from build123d import *

# Parameters (mm, degrees)
SKETCH1_R           = 5
BOSS_EXTRUDE1_DEPTH = 6
BOSS_EXTRUDE2_DEPTH = 3
SKETCH3_R           = 3
SKETCH3_R_2         = 1.25
CUT_EXTRUDE1_DEPTH  = 14.865424624
FILLET1_R           = 0.3
CHAMFER1_SIZE       = 0.1


with BuildPart() as part:
    # Sketch1 → Boss-Extrude1 (new body)
    with BuildSketch(Plane.XY):
        Circle(SKETCH1_R)
    extrude(amount=BOSS_EXTRUDE1_DEPTH)

    # Sketch2 → Boss-Extrude2 (add)
    with BuildSketch(Plane(origin=(0, 0, 0), x_dir=(-1, 0, 0), z_dir=(0, 0, -1))):
        with BuildLine():
            Line((-4.763139721, 2.75), (-1.732050808, 8))
            ThreePointArc((-1.732050808, 8), (0, 9), (1.732050808, 8))
            Line((1.732050808, 8), (4.763139721, 2.75))
            ThreePointArc((4.763139721, 2.75), (5.5, 0), (4.763139721, -2.75))
            Line((4.763139721, -2.75), (1.732050808, -8))
            ThreePointArc((1.732050808, -8), (0, -9), (-1.732050808, -8))
            Line((-1.732050808, -8), (-4.763139721, -2.75))
            ThreePointArc((-4.763139721, -2.75), (-5.5, 0), (-4.763139721, 2.75))
        make_face()
    extrude(amount=BOSS_EXTRUDE2_DEPTH)

    # Sketch3 → Cut-Extrude1 (cut, through all)
    with BuildSketch(Plane(origin=(0, 0, -3), x_dir=(-1, 0, 0), z_dir=(0, 0, -1))):
        Circle(SKETCH3_R)
        with Locations((0, 7)):
            Circle(SKETCH3_R_2)
        with Locations((0, -7)):
            Circle(SKETCH3_R_2)
    extrude(amount=-CUT_EXTRUDE1_DEPTH, mode=Mode.SUBTRACT)

    # Fillet1
    fillet1_edges = [part.edges().sort_by_distance(p)[0] for p in [
        (-5, 0, 0),
    ]]
    fillet(fillet1_edges, radius=FILLET1_R)

    # Chamfer1
    chamfer1_edges = [part.edges().sort_by_distance(p)[0] for p in [
        (-3.247595264, -5.375, -3),
        (-5.5, 0, -3),
        (-3.247595264, 5.375, -3),
        (0, 9, -3),
        (3.247595264, 5.375, -3),
        (1.25, -7, 0),
        (1.25, -7, -3),
        (1.25, 7, 0),
        (1.25, 7, -3),
        (3, 0, 6),
        (3, 0, -3),
        (-5, 0, 6),
        (5.5, 0, 0),
        (3.247595264, -5.375, 0),
        (0, -9, 0),
        (-3.247595264, -5.375, 0),
        (-5.5, 0, 0),
        (-3.247595264, 5.375, 0),
        (0, 9, 0),
        (3.247595264, 5.375, 0),
        (5.5, 0, -3),
        (3.247595264, -5.375, -3),
        (0, -9, -3),
    ]]
    chamfer(chamfer1_edges, length=CHAMFER1_SIZE)


solid = part.part
Part model, mm, in its own coordinate system. A direction names the side the tool comes from. Coordinates: 2 decimals unless noted, no trailing zeros. Loops run counter-clockwise (first coordinate to the right, second up) from the corner with the lowest first, then second, coordinate; pieces in that order, holes last. Notation, with made-up numbers: M 76,65 L 96,65 A29 cw 96,102 Z; hole C -5.5,85 d11. An arc over 180 degrees is marked long. Use a Markdown table: item, result. Add a question column.
Q1. Probe L1, parallel to Y at x = 0, z = 3; L2, parallel to Z at x = -2.25, y = 5.25; L3, parallel to Y at x = -1, z = -0.5. List the from-to ranges inside material, lowest first.
Q2. Pin check, flat tips, straight feed: P1, Ø3, axis at x = -2.5, z = 3.5, coming from the -Y side; P2, Ø4, axis at x = -4, y = -7, coming from the +Z side; P3, Ø2, axis at x = 3, z = 4.5, coming from the -Y side. Stop position of each tip, or through.
Q3. Cut at B-B (z = -2). Write the cut outline in (x, y), and give its area (3 significant figures).
Q4. Cut at D-D (x = 0). Give the number of separate pieces and of enclosed holes in the cut face, and give its area (3 significant figures).
Q5. Which spindle directions (+Z, -Z, +X, -X, +Y, -Y) get a long thin tool onto all of the face, cutting with end or side? Do faces 1 (the flat face through (3.226, -5.412, -1.48)), 2 (the cylindrical face through (-1.08, -4.88, 3.06)). Say none if no direction does.
Q6. Cut at C-C (z = 3.75). Write the cut outline in (x, y).
Q7. Cut at A-A (y = 0). Write the cut outline in (x, z), and give its area (3 significant figures).
Q8. Mould opens along Y. For faces 3 (the cylindrical face through (0.27, 5.78, -1.52)), 4 (the cylindrical face through (-5.5, 0, -1.5)), 5 (the flat face through (-3.27, -5.34, -1.48)) say: +Y half, -Y half, draft (parallel to the pull), parting line (faces both ways), or undercut.
Worked out:
| question | item | result |
|---|---|---|
| 1 | L1 | y = -5 to -3, 3 to 5 |
| 1 | L2 | z = -3 to 0 |
| 1 | L3 | y = -8.73 to -7.75, -6.25 to -2.83, 2.83 to 6.25, 7.75 to 8.73 |
| 2 | P1 | stops at y = -4.9 |
| 2 | P2 | stops at z = 0 |
| 2 | P3 | stops at y = -4.58 |
| 3 | outline | M -4.76,-2.75 L -1.73,-8 A2 ccw 1.73,-8 L 4.76,-2.75 A5.5 ccw 4.76,2.75 L 1.73,8 A2 ccw -1.73,8 L -4.76,2.75 A5.5 ccw Z; hole C 0,0 d6; hole C 0,-7 d2.5; hole C 0,7 d2.5 |
| 3 | area | 92.9 mm2 |
| 4 | separate pieces | 4 |
| 4 | enclosed holes | 0 |
| 4 | area | 44.9 mm2 |
| 5 | face 1 | +Z, -Z, +X, -Y |
| 5 | face 2 | +Z |
| 6 | outline | C 0,0 d10; hole C 0,0 d6 |
| 7 | outline | M -5.5,-2.9 L -5.4,-3 L -3.1,-3 L -3,-2.9 L -3,5.9 L -3.1,6 L -4.9,6 L -5,5.9 L -5,0.3 A0.3 cw -5.3,0 L -5.4,0 L -5.5,-0.1 Z; M 3,-2.9 L 3.1,-3 L 5.4,-3 L 5.5,-2.9 L 5.5,-0.1 L 5.4,0 L 5.3,0 A0.3 cw 5,0.3 L 5,5.9 L 4.9,6 L 3.1,6 L 3,5.9 Z |
| 7 | area | 39.0 mm2 |
| 8 | face 3 | undercut |
| 8 | face 4 | parting line |
| 8 | face 5 | -Y half |
